```python
from build123d import *

# Parameters (mm, degrees)
SKETCH_1_R          = 2.05
SKETCH_1_R_2        = 1.05
EXTRUDE_1_DEPTH     = 7.5
FILLET_1_R          = 0.2
SKETCH_2_R          = 3.05
CUT_EXTRUDE_1_DEPTH = 1


with BuildPart() as part:
    # 草图1 → 凸台-拉伸1 (new body)
    with BuildSketch(Plane(origin=(0, 0, 0), x_dir=(1, 0, 0), z_dir=(0, 1, 0))):
        Circle(SKETCH_1_R)
        Circle(SKETCH_1_R_2, mode=Mode.SUBTRACT)
    extrude(amount=EXTRUDE_1_DEPTH)

    # 圆角1
    fillet_1_edges = [part.edges().sort_by_distance(p)[0] for p in [
        (-2.05, 0, 0),
        (-2.05, 7.5, 0),
        (-1.05, 0, 0),
        (-1.05, 7.5, 0),
    ]]
    fillet(fillet_1_edges, radius=FILLET_1_R)

    # 草图2 → 切除-拉伸1 (cut)
    with BuildSketch(Plane(origin=(0, 7.5, 0), x_dir=(1, 0, 0), z_dir=(0, 1, 0))):
        Circle(SKETCH_2_R)
    extrude(amount=-CUT_EXTRUDE_1_DEPTH, mode=Mode.SUBTRACT)


solid = part.part
```
Source: CAD feature listing. Evaluate the final solid. Frame: model axes, mm. Give positions to 0.01 mm unless a question says otherwise; leave off trailing zeros. Write each loop counter-clockwise with the first axis right and the second up, starting at its lowest first coordinate (ties: lowest second). Pieces come first, ordered by that corner, then holes. Notation, with made-up numbers: (23, -32) - (60, -32) arc R20 ccw to (60, -27) - close; hole circle Ø2 at (-28.75, 52.5). An arc over 180 degrees is marked (long way). One line per item, written item: value. Start each with the question number.
Q1. Section query B-B, the plane z = 0. Return the cut outline in (x, y), then the cut area to 3 significant figures.
Q2. First-contact query: pin 1 Ø2 at (y, z) = (3.5, -0.5) entering from +X; pin 2 Ø1 at (x, y) = (-1, 5.5) entering from -Z. Flat tips, straight axial feed; report the tip coordinate or a pass-through.
Q3. Material intervals for probe 1 along X at (y, z) = (2.75, 0); probe 2 along X at (y, z) = (4, -0.7); probe 3 along Z at (x, y) = (0.65, 3.5), sorted ascending. Write a range as from..to.
Q4. Section query A-A, the plane x = 0. Return the cut outline in (y, z), then the cut area to 3 significant figures.
Q5. Section query C-C, the plane y = 4.25. Return the cut outline in (x, z), then the cut area to 3 significant figures.
Q6. Draft query along X for faces 1 (the face through (1, 6.5, 1)), 2 (the face through (-0.267, 3.306, -2.033)), 3 (the face through (1, 3.31, -0.32)). Return one class per face: +X half, -X half, draft (parallel to the pull), parting line (faces both ways), or undercut.
Answer:
1. outline: (-2.05, 0.2) arc R0.2 ccw to (-1.85, 0) - (-1.25, 0) arc R0.2 ccw to (-1.05, 0.2) - (-1.05, 6.5) - (-2.05, 6.5) - close; (1.05, 0.2) arc R0.2 ccw to (1.25, 0) - (1.85, 0) arc R0.2 ccw to (2.05, 0.2) - (2.05, 6.5) - (1.05, 6.5) - close
1. area: 13.0 mm2
2. pin 1: stops at x = 2.05
2. pin 2: stops at z = -1.99
3. probe 1: x = -2.05..-1.05, 1.05..2.05
3. probe 2: x = -1.93..-0.78, 0.78..1.93
3. probe 3: z = -1.94..-0.82, 0.82..1.94
4. outline: (0, -1.85) arc R0.2 ccw to (0.2, -2.05) - (6.5, -2.05) - (6.5, -1.05) - (0.2, -1.05) arc R0.2 ccw to (0, -1.25) - close; (0, 1.25) arc R0.2 ccw to (0.2, 1.05) - (6.5, 1.05) - (6.5, 2.05) - (0.2, 2.05) arc R0.2 ccw to (0, 1.85) - close
4. area: 13.0 mm2
5. outline: circle Ø4.1 at (0, 0); hole circle Ø2.1 at (0, 0)
5. area: 9.74 mm2
6. face 1: draft
6. face 2: parting line
6. face 3: undercut
